```python
from build123d import *

# Parameters (mm, degrees)
F0_W     = 122.2604140639
F0_H     = 78.6352567375
F2_DEPTH = 25.4
F3_T     = -2.54
F1_W     = 63.6047422886
F1_H     = 78.8185559213
F4_DEPTH = 5.588
F5_R     = 1.6394762834
F6_DEPTH = 28.194
F5_R_2   = 1.6394765438
F7_DEPTH = 32.258


# Not quite as in the source:
# - the program builds the solid bodies; features that only make, move or delete a surface that nothing else refers to are left out


with BuildPart() as f2:
    # F0 (on Top) → F2 (new body)
    with BuildSketch(Plane.XY):
        with BuildLine():
            ThreePointArc((63.7880414724, 35.6516502798), (2.6578344405, 42.8155765092), (-58.4723725915, 35.6516502798))
            Line((-58.4723725915, 35.6516502798), (63.7880414724, 35.6516502798))
        make_face()
        with Locations((2.6578344405, -3.665978089)):
            Rectangle(F0_W, F0_H)
        with BuildLine():
            Line((63.7880414724, -42.9836064577), (-58.4723725915, -42.9836064577))
            ThreePointArc((-58.4723725915, -42.9836064577), (2.6578344405, -50.1645132958), (63.7880414724, -42.9836064577))
        make_face()
    extrude(amount=F2_DEPTH)

    # F3
    f3_openings = [f2.faces().sort_by_distance(p)[0] for p in [
        (-58.472373, -3.665978, 12.7),
    ]]
    offset(amount=F3_T, openings=f3_openings)

    # F1 (on Top) → F4 (join)
    with BuildSketch(Plane.XY):
        with Locations((31.8023711443, -3.7576276809)):
            Rectangle(F1_W, F1_H)
    extrude(amount=F4_DEPTH)

    # F5 (on Front) → F6 (cut)
    with BuildSketch(Plane.XZ):
        with Locations((-47.8410311043, 4.857422784)):
            Circle(F5_R)
    extrude(amount=-F6_DEPTH, mode=Mode.SUBTRACT)

    # F5 (on Front) → F7 (cut)
    with BuildSketch(Plane.XZ):
        with Locations((-13.1975244731, 4.857422784)):
            Circle(F5_R_2)
        with Locations((-47.8410311043, 4.857422784)):
            Circle(F5_R)
    extrude(amount=-F7_DEPTH, mode=Mode.SUBTRACT)


solid = f2.part
```
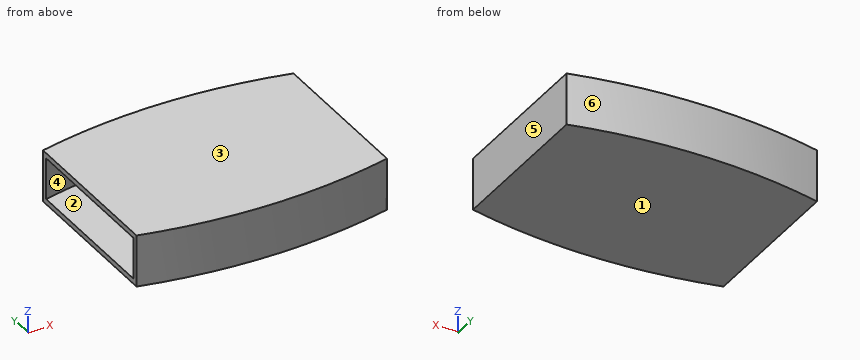
Work out the finished part from the listing and answer in its coordinate system (mm). Face numbers are marked on the shaded views. A direction names the side the tool comes from. Give positions to 0.01 mm unless a question says otherwise; leave off trailing zeros. Write each loop counter-clockwise with the first axis right and the second up, starting at its lowest first coordinate (ties: lowest second). Pieces come first, ordered by that corner, then holes. Notation, with made-up numbers: (39, 13) - (50, 13) arc R19 cw to (50, 26) - close; hole circle Ø5 at (87, 27.25). An arc over 180 degrees is marked (long way). Use one line per item in the form item = value.
1. Each of these flat-tipped pins is pushed along its axis until it touches: pin 1 Ø3 at (x, z) = (39.5, 11.5) entering from -Y; pin 2 Ø8.5 at (y, z) = (8, 18.5) entering from -X; pin 3 Ø3.5 at (x, z) = (28, 4.5) entering from -Y. Where does it stop, or does it pass through?
Filled in:
pin_1 = -47.79
pin_2 = 61.25
pin_3 = -49.11
2. A cutting plane is placed at B-B (y = 9.5). Write down the section's boundary in (x, z), and give its area (3 significant figures).
Filled in:
outline = (-58.47, 0) - (63.79, 0) - (63.79, 25.4) - (-58.47, 25.4) - (-58.47, 22.86) - (61.25, 22.86) - (61.25, 5.59) - (0, 5.59) - (0, 2.54) - (-58.47, 2.54) - close
area = 859 mm^2
3. Consider L1, parallel to Z at x = 40, y = 0.5; L2, parallel to Y at x = 10, z = 4.25; L3, parallel to Z at x = -37, y = -1.5. Determine where each line is inside the solid, lowest interval first.
Filled in:
L1 = 0 to 5.59, 22.86 to 25.4
L2 = -50.06 to -47.52, -43.17 to 35.65, 40.17 to 42.71
L3 = 0 to 2.54, 22.86 to 25.4
4. Determine the mould class of the marked faces 3, 4, 5 and 6 for opening direction X: released by +X, released by -X, zero draft, split by the parting line, or undercut.
Filled in:
face_3 = zero draft
face_4 = undercut
face_5 = released by +X
face_6 = split by the parting line
5. A cutting plane is placed at C-C (z = 7). Write down the section's boundary in (x, y).
Filled in:
outline = (-58.47, -42.98) arc R263.79 ccw to (63.79, -42.98) - (63.79, 35.65) arc R264.4 ccw to (-58.47, 35.65) - (-58.47, 33.04) arc R261.86 cw to (61.25, 33.64) - (61.25, -40.97) arc R261.25 cw to (-58.47, -40.37) - close
6. For the marked faces 1 and 2, determine the directions among +Z, -Z, +X, -X, +Y, -Y from which every point of the face is accessible in a straight line to the end or side of a thin tool.
Filled in:
face_1 = -Z, +X, -X, +Y, -Y
face_2 = none
7. A cutting plane is placed at A-A (x = 21). Write down the section's boundary in (y, z).
Filled in:
outline = (-49.53, 0) - (42.18, 0) - (42.18, 25.4) - (-49.53, 25.4) - close; hole (-46.98, 2.54) - (-43.17, 2.54) - (-43.17, 5.59) - (35.65, 5.59) - (35.65, 2.54) - (39.63, 2.54) - (39.63, 22.86) - (-46.98, 22.86) - close
8. A cutting plane is placed at D-D (x = -9.5). Write down the section's boundary in (y, z).
Filled in:
outline = (-49.88, 0) - (42.54, 0) - (42.54, 25.4) - (-49.88, 25.4) - close; hole (-47.34, 2.54) - (39.99, 2.54) - (39.99, 22.86) - (-47.34, 22.86) - close
